from build123d import *

# Parameters (mm, degrees)
BOSS_EXTRUDE1_DEPTH = 55
BOSS_EXTRUDE2_DEPTH = 6.5


with BuildPart() as part:
    # Sketch1 → Boss-Extrude1 (new, symmetric)
    with BuildSketch(Plane.XY):
        with BuildLine():
            Line((5, 29.580398915), (5, 39.686269666))
            ThreePointArc((5, 39.686269666), (40, 0), (5, -39.686269666))
            Line((5, -39.686269666), (5, -29.580398915))
            ThreePointArc((5, -29.580398915), (30, 0), (5, 29.580398915))
        make_face()
    extrude(amount=BOSS_EXTRUDE1_DEPTH, both=True)

    # Sketch2 → Boss-Extrude2 (add, symmetric)
    with BuildSketch(Plane.XY.offset(55)):
        with BuildLine():
            Line((5, 29.580398915), (5, 47.236109069))
            ThreePointArc((5, 47.236109069), (47.5, 0), (5, -47.236109069))
            Line((5, -47.236109069), (5, -29.580398915))
            ThreePointArc((5, -29.580398915), (30, 0), (5, 29.580398915))
        make_face()
    boss_extrude2 = extrude(amount=BOSS_EXTRUDE2_DEPTH, both=True)

    # Mirror2: Boss-Extrude2 across plane
    add(boss_extrude2.mirror(Plane.XY))


solid = part.part
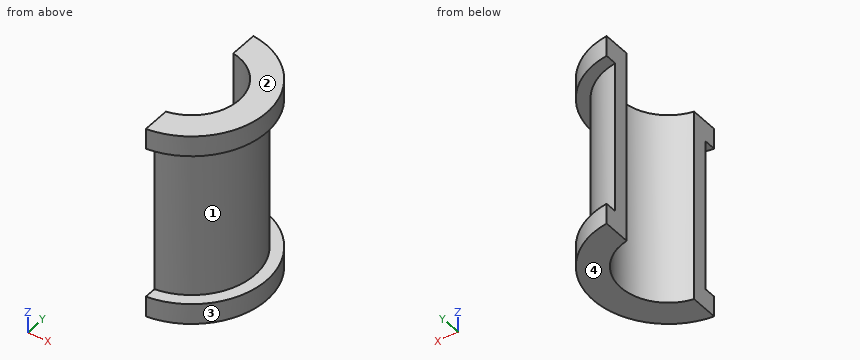
Geometry: final body of the model. Coordinates: model frame, mm. Face numbers are marked on the shaded views. Give positions to 0.01 mm unless a question says otherwise; leave off trailing zeros. Loops run counter-clockwise (first coordinate to the right, second up) from the corner with the lowest first, then second, coordinate; pieces in that order, holes last. Notation, with made-up numbers: M 7.25,58.25 L 33.25,58.25 A26 cw 33.25,86.25 Z; hole C 64,-23.75 d4. An arc over 180 degrees is marked long. Put each result on its own line as item: value.
1) Cut plane C-C, the plane y = -4.5. Return the cut outline in (x, z), plus the area to 3 significant figures.
Computed values:
outline: M 29.66,-61.5 L 47.29,-61.5 L 47.29,-48.5 L 39.75,-48.5 L 39.75,48.5 L 47.29,48.5 L 47.29,61.5 L 29.66,61.5 Z
area: 1,440 mm^2
2) First-contact query: P1, Ø8, axis at x = 13.5, z = -44, coming from the -Y side; P2, Ø13, axis at x = 19.5, y = 0.5, coming from the +Z side; P3, Ø4, axis at x = 19, z = 42, coming from the +Y side; P4, Ø1, axis at y = 22.5, z = -3, coming from the -X side. Flat tips, straight axial feed; report the tip coordinate or a pass-through.
Computed values:
P1: stops at y = -38.86
P2: passes through
P3: stops at y = 36.21
P4: stops at x = 19.26
3) Cut plane D-D, the plane x = 12.5. Return the cut outline in (y, z), plus the area to 3 significant figures.
Computed values:
outline: M -45.83,-61.5 L -27.27,-61.5 L -27.27,61.5 L -45.83,61.5 L -45.83,48.5 L -38,48.5 L -38,-48.5 L -45.83,-48.5 Z; M 27.27,-61.5 L 45.83,-61.5 L 45.83,-48.5 L 38,-48.5 L 38,48.5 L 45.83,48.5 L 45.83,61.5 L 27.27,61.5 Z
area: 3,050 mm^2
4) Cut plane A-A, the plane x = 38. Return the cut outline in (y, z), plus the area to 3 significant figures.
Computed values:
outline: M -28.5,-61.5 L 28.5,-61.5 L 28.5,-48.5 L 12.49,-48.5 L 12.49,48.5 L 28.5,48.5 L 28.5,61.5 L -28.5,61.5 L -28.5,48.5 L -12.49,48.5 L -12.49,-48.5 L -28.5,-48.5 Z
area: 3,910 mm^2
5) Material intervals for L1, parallel to Z at x = 38, y = -13; L2, parallel to Y at x = 9, z = 46.5; L3, parallel to Y at x = 13, z = -26.5, sorted ascending. Write a range as from..to.
Computed values:
L1: z = -61.5..-48.5, 48.5..61.5
L2: y = -38.97..-28.62, 28.62..38.97
L3: y = -37.83..-27.04, 27.04..37.83
6) Cut plane B-B, the plane x = 44.5. Return the cut outline in (y, z).
Computed values:
outline: M -16.61,-61.5 L 16.61,-61.5 L 16.61,-48.5 L -16.61,-48.5 Z; M -16.61,48.5 L 16.61,48.5 L 16.61,61.5 L -16.61,61.5 Z
7) Mould query, pull axis Z, two halves, no side actions, for the marked faces 1, 2, 3 and 4. Classes: released by +Z, released by -Z, zero draft, split by the parting line, or undercut.
Computed values:
face 1: undercut
face 2: released by +Z
face 3: zero draft
face 4: released by -Z
